CAD build for the part. Positions are in the model's coordinates, mm. Face numbers are marked on the shaded views. A direction names the side the tool comes from. Give positions to 0.01 mm unless a question says otherwise; leave off trailing zeros. Loops run counter-clockwise (first coordinate to the right, second up) from the corner with the lowest first, then second, coordinate; pieces in that order, holes last. Notation, with made-up numbers: (17.25, -18.75) -> (55.25, -18.75) arc R5 cw to (55.25, -14.75) -> close; hole circle Ø6 at (68, 66). An arc over 180 degrees is marked (long way). Use one line per item in the form item = value.
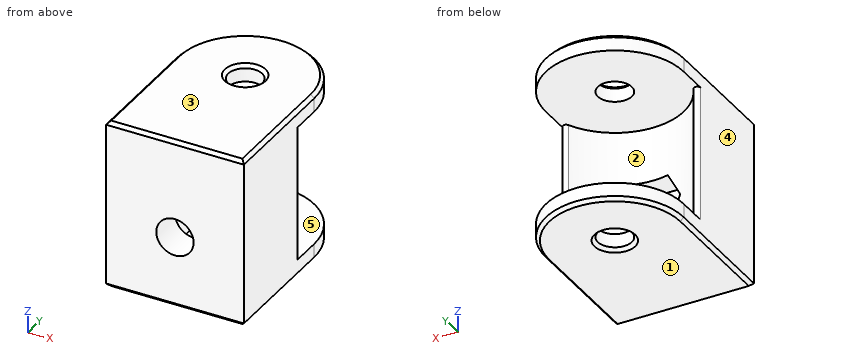
```python
from build123d import *

# Parameters (mm, degrees)
SKETCH1_W               = 20.32
SKETCH1_H               = 25
BOSS_EXTRUDE1_DEPTH     = 28.82
SKETCH2_W               = 20
SKETCH2_H               = 20.32
CUT_EXTRUDE1_DEPTH      = 38.413163459
SKETCH3_R               = 2.5
CUT_EXTRUDE2_DEPTH      = 28.82
BOSS_EXTRUDE2_START     = 20
BOSS_EXTRUDE2_DEPTH     = 20
FILLET1_START           = -10
FILLET1_DEPTH           = 20
CUT_EXTRUDE3_DEPTH      = 34.016177853
CUT_EXTRUDE3_DEPTH_BACK = 3.5
CUT_EXTRUDE3_START      = 8.5
SKETCH5_R               = 2.75
CUT_EXTRUDE4_DEPTH      = 29.755312553
CHAMFER1_SIZE           = 0.5


with BuildPart() as part:
    # Sketch1 → Boss-Extrude1 (new body)
    with BuildSketch(Plane(origin=(0, 0, 0), x_dir=(1, 0, 0), z_dir=(0, 1, 0))):
        Rectangle(SKETCH1_W, SKETCH1_H)
    extrude(amount=BOSS_EXTRUDE1_DEPTH)

    # Sketch2 → Cut-Extrude1 (cut, through all)
    with BuildSketch(Plane(origin=(10.16, 0, 0), x_dir=(0, 0, -1), z_dir=(1, 0, 0))):
        with Locations((0, 18.66)):
            Rectangle(SKETCH2_W, SKETCH2_H)
    extrude(amount=-CUT_EXTRUDE1_DEPTH, mode=Mode.SUBTRACT)

    # Sketch3 → Cut-Extrude2 (cut)
    with BuildSketch(Plane.XY.offset(12.5)):
        with Locations((0, 18.66)):
            Circle(SKETCH3_R)
        with BuildLine():
            Line((-10.16, 18.66), (-10.16, 30.66))
            Line((-10.16, 30.66), (10.16, 30.66))
            Line((10.16, 30.66), (10.16, 18.66))
            ThreePointArc((10.16, 18.66), (0, 28.82), (-10.16, 18.66))
        make_face()
    extrude(amount=-CUT_EXTRUDE2_DEPTH, mode=Mode.SUBTRACT)

    # Sketch7 → Boss-Extrude2 (add)
    with BuildSketch(Plane.XY.offset(-10).offset(BOSS_EXTRUDE2_START)):
        with BuildLine():
            Line((10.16, 18.66), (10.16, 0))
            Line((10.16, 0), (-10.16, 0))
            Line((-10.16, 0), (-10.16, 18.66))
            ThreePointArc((-10.16, 18.66), (0, 8.5), (10.16, 18.66))
        make_face()
    extrude(amount=-BOSS_EXTRUDE2_DEPTH)

    # Fillet1: read off the stored shape, not the designer's step
    # Fillet1 outline → Fillet1 (cut)
    with BuildSketch(Plane.XY.offset(FILLET1_START)):
        with BuildLine():
            ThreePointArc((10.16, 18.66), (9.918864548, 16.459607744), (9.206904315, 14.363662847))
            ThreePointArc((9.206904315, 14.363662847), (9.76828702, 14.64036203), (10.16, 14.152228932))
            Line((10.16, 14.152228932), (10.16, 18.66))
        make_face()
        with BuildLine():
            ThreePointArc((-10.16, 14.152228932), (-9.76828702, 14.64036203), (-9.206904315, 14.363662847))
            ThreePointArc((-9.206904315, 14.363662847), (-9.918864548, 16.459607744), (-10.16, 18.66))
            Line((-10.16, 18.66), (-10.16, 14.152228932))
        make_face()
    extrude(amount=FILLET1_DEPTH, mode=Mode.SUBTRACT)

    # Sketch4 → Cut-Extrude3 (cut, two sides: drawn at the far end of the back side and taken through both)
    with BuildSketch(Plane(origin=(0, 0, 0), x_dir=(1, 0, 0), z_dir=(0, 1, 0)).offset(CUT_EXTRUDE3_START - CUT_EXTRUDE3_DEPTH_BACK)):
        Polygon((4.618802154, 2), (2.309401077, 6), (-2.309401077, 6), (-4.618802154, 2), (-2.309401077, -2), (2.309401077, -2), align=None)
    extrude(amount=CUT_EXTRUDE3_DEPTH + CUT_EXTRUDE3_DEPTH_BACK, mode=Mode.SUBTRACT)

    # Sketch5 → Cut-Extrude4 (cut, through all)
    with BuildSketch(Plane(origin=(0, 5, 0), x_dir=(1, 0, 0), z_dir=(0, 1, 0))):
        with Locations(Location((0, 2, 0), (0, 0, 270))):
            Circle(SKETCH5_R)
    extrude(amount=-CUT_EXTRUDE4_DEPTH, mode=Mode.SUBTRACT)

    # Chamfer1
    chamfer1_edges = [part.edges().sort_by_distance(p)[0] for p in [
        (10.16, 9.33, 12.5),
        (-10.16, 9.33, 12.5),
        (-10.16, 9.33, -12.5),
        (10.16, 9.33, -12.5),
        (-2.5, 18.66, -12.5),
        (-2.5, 18.66, 12.5),
        (0, 28.82, 12.5),
        (0, 28.82, -12.5),
        (0, 0, 12.5),
        (0, 0, -12.5),
    ]]
    chamfer(chamfer1_edges, length=CHAMFER1_SIZE)


solid = part.part
```
1. Cut at A-A, the plane y = 2. Write the cut outline in (x, z), then the cut area to 3 significant figures.
Result sheet:
outline = (-10.16, -12) -> (-9.66, -12.5) -> (9.66, -12.5) -> (10.16, -12) -> (10.16, 12) -> (9.66, 12.5) -> (-9.66, 12.5) -> (-10.16, 12) -> close; hole circle Ø5.5 at (0, -2)
area = 484 mm^2
2. Cut at D-D, the plane y = 7. Write the cut outline in (x, z), then the cut area to 3 significant figures.
Result sheet:
outline = (-10.16, -12) -> (-9.66, -12.5) -> (9.66, -12.5) -> (10.16, -12) -> (10.16, 12) -> (9.66, 12.5) -> (-9.66, 12.5) -> (-10.16, 12) -> close; hole (-4.62, -2) -> (-2.31, -6) -> (2.31, -6) -> (4.62, -2) -> (2.31, 2) -> (-2.31, 2) -> close
area = 452 mm^2
3. Drop flat-ended pins along their axis: P1, Ø9, axis at x = 0, z = -2, coming from the +Y side; P2, Ø4, axis at x = 1.5, z = -5, coming from the +Y side; P3, Ø10, axis at x = -1.5, z = -1, coming from the +Y side. Give the stop position or say it passes through.
Result sheet:
P1 = 9.55
P2 = 9.12
P3 = 10.85
4. Cut at B-B, the plane x = 0. State how many separate pieces and enclosed holes the cut face has, then the cut area to 3 significant figures.
Result sheet:
separate_pieces = 4
enclosed_holes = 0
area = 233 mm^2
5. Cut at C-C, the plane z = -1. Write the cut outline in (x, y).
Result sheet:
outline = (-10.16, 0) -> (-2.56, 0) -> (-2.56, 5) -> (-4.04, 5) -> (-4.04, 9.34) arc R10.16 cw to (-9.21, 14.36) arc R0.5 ccw to (-10.16, 14.15) -> close; (2.56, 0) -> (10.16, 0) -> (10.16, 14.15) arc R0.5 ccw to (9.21, 14.36) arc R10.16 cw to (4.04, 9.34) -> (4.04, 5) -> (2.56, 5) -> close
6. Drill centre lines: line 1 (Y direction, x = 0, z = 11.3); line 2 (Z direction, x = 2, y = 21.5); line 3 (X direction, y = 3.4, z = -2). Where is each one in solid material? Low to high.
Result sheet:
line_1 = 0 to 16.16, 21.16 to 28.82
line_2 = -12.5 to -10, 10 to 12.5
line_3 = -10.16 to -2.75, 2.75 to 10.16
7. Mould opens along Z. For the marked faces 3, 4 and 5 say: pulls with the +Z half, pulls with the -Z half, needs draft (parallel to the pull), parting line crosses it, or undercut.
Result sheet:
face_3 = pulls with the +Z half
face_4 = needs draft
face_5 = undercut
8. Tool access for the marked faces 1 and 2: list every direction of +Z, -Z, +X, -X, +Y, -Y with a clear straight run to the whole face (end or side of a thin tool).
Result sheet:
face_1 = -Z, +X, -X, +Y, -Y
face_2 = +Y
